Geometry: final body of the model. Coordinates: model frame, mm. Coordinates: 2 decimals unless noted, no trailing zeros. Loops run counter-clockwise (first coordinate to the right, second up) from the corner with the lowest first, then second, coordinate; pieces in that order, holes last. Notation, with made-up numbers: (-33.5, 30) -> (-25.5, 30) arc R18 cw to (-25.5, 45) -> close; hole circle Ø6 at (82, 67). An arc over 180 degrees is marked (long way). One line per item, written item: value. Start each with the question number.
from build123d import *

# Parameters (mm, degrees)
SKETCH1_W           = 77
SKETCH1_H           = 65
BOSS_EXTRUDE1_DEPTH = 3
SKETCH2_R           = 2.75
CUT_EXTRUDE1_DEPTH  = 109.935760887
SKETCH3_R           = 1.65
SKETCH3_R_2         = 9.6
CUT_EXTRUDE2_DEPTH  = 109.935760887
FILLET1_R           = 10
SKETCH4_W           = 77
SKETCH4_H           = 6
BOSS_EXTRUDE2_DEPTH = 3
SKETCH5_R           = 2
CUT_EXTRUDE3_DEPTH  = 109.935760887
SKETCH6_R           = 8
SKETCH6_R_2         = 2.5
CUT_EXTRUDE4_DEPTH  = 109.935760887


with BuildPart() as part:
    # Sketch1 → Boss-Extrude1 (new body)
    with BuildSketch(Plane.XY):
        with Locations((38.5, 44.5)):
            Rectangle(SKETCH1_W, SKETCH1_H)
        Polygon((77, 12), (38.5, 12), (38.5, 0), (77, 0), (77, 3), (71, 3), (71, 9), (77, 9), align=None)
        Polygon((38.5, 0), (38.5, 12), (0, 12), (0, 9), (6, 9), (6, 3), (0, 3), (0, 0), align=None)
    extrude(amount=BOSS_EXTRUDE1_DEPTH)

    # Sketch2 → Cut-Extrude1 (cut, through all)
    with BuildSketch(Plane.XY.offset(3)):
        with Locations((21, 6)):
            Circle(SKETCH2_R)
        with Locations((56, 6)):
            Circle(SKETCH2_R)
    extrude(amount=-CUT_EXTRUDE1_DEPTH, mode=Mode.SUBTRACT)

    # Sketch3 → Cut-Extrude2 (cut, through all)
    with BuildSketch(Plane.XY.offset(3)):
        with Locations((29.307611845, 46.807611845)):
            Circle(SKETCH3_R)
        with Locations((47.692388155, 46.807611845)):
            Circle(SKETCH3_R)
        with Locations((47.692388155, 65.192388155)):
            Circle(SKETCH3_R)
        with Locations((29.307611845, 65.192388155)):
            Circle(SKETCH3_R)
        with Locations((38.5, 56)):
            Circle(SKETCH3_R_2)
    extrude(amount=-CUT_EXTRUDE2_DEPTH, mode=Mode.SUBTRACT)

    # Fillet1
    fillet1_edges = [part.edges().sort_by_distance(p)[0] for p in [
        (0, 77, 1.5),
        (77, 77, 1.5),
    ]]
    fillet(fillet1_edges, radius=FILLET1_R)

    # Sketch4 → Boss-Extrude2 (add)
    with BuildSketch(Plane.XY.offset(3)):
        with Locations((38.5, -3)):
            Rectangle(SKETCH4_W, SKETCH4_H)
    extrude(amount=-BOSS_EXTRUDE2_DEPTH)

    # Sketch5 → Cut-Extrude3 (cut, through all)
    with BuildSketch(Plane.XY.offset(3)):
        with Locations((8, -1.5)):
            Circle(SKETCH5_R)
        with Locations((69, -1.5)):
            Circle(SKETCH5_R)
        with Locations((8, 18)):
            Circle(SKETCH5_R)
        with Locations((69, 18)):
            Circle(SKETCH5_R)
    extrude(amount=-CUT_EXTRUDE3_DEPTH, mode=Mode.SUBTRACT)

    # Sketch6 → Cut-Extrude4 (cut, through all)
    # profile 1 of 2: a face of its own
    with BuildSketch(Plane.XY.offset(3)):
        with Locations((65, 56)):
            Circle(SKETCH6_R)
        with Locations((65, 56)):
            Circle(SKETCH6_R_2, mode=Mode.SUBTRACT)
    # profile 2 of 2: a face of its own
    with BuildSketch(Plane.XY.offset(3)):
        with Locations((65, 56)):
            Circle(SKETCH6_R_2)
    extrude(amount=-CUT_EXTRUDE4_DEPTH, mode=Mode.SUBTRACT)


solid = part.part
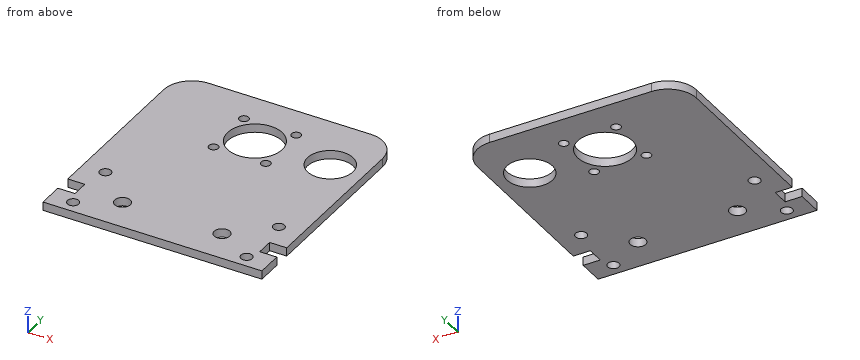
1. Section B-B on y = 18. Return the cut outline in (x, z).
2. Section D-D on x = 56. Return the cut outline in (y, z).
3. Line query: L1, parallel to Y at x = 21, z = 0.6; L2, parallel to X at y = 18.5, z = 0.75; L3, parallel to X at y = 66, z = 1.3. Output: solid intervals per line, ascending. Write a range as [from, to].
4. Section A-A on x = 65. Return the cut outline in (y, z), plus the area to 3 significant figures.
5. Pin query (flat end, axial travel): pin 1 Ø1.5 at (x, z) = (74, 1.5) entering from +Y; pin 2 Ø0.9 at (x, z) = (2, 2) entering from +Y. Return the tip coordinate at first contact, or that it passes through.
Checks:
1. outline: (0, 0) -> (6, 0) -> (6, 3) -> (0, 3) -> close; (10, 0) -> (67, 0) -> (67, 3) -> (10, 3) -> close; (71, 0) -> (77, 0) -> (77, 3) -> (71, 3) -> close
2. outline: (-6, 0) -> (3.25, 0) -> (3.25, 3) -> (-6, 3) -> close; (8.75, 0) -> (77, 0) -> (77, 3) -> (8.75, 3) -> close
3. L1: [-6, 3.25], [8.75, 77]
3. L2: [0, 6.06], [9.94, 67.06], [70.94, 77]
3. L3: [0, 27.87], [30.75, 46.25], [49.13, 77]
4. outline: (-6, 0) -> (48, 0) -> (48, 3) -> (-6, 3) -> close; (64, 0) -> (77, 0) -> (77, 3) -> (64, 3) -> close
4. area: 201 mm²
5. pin 1: y = 74.81
5. pin 2: y = 73.56
